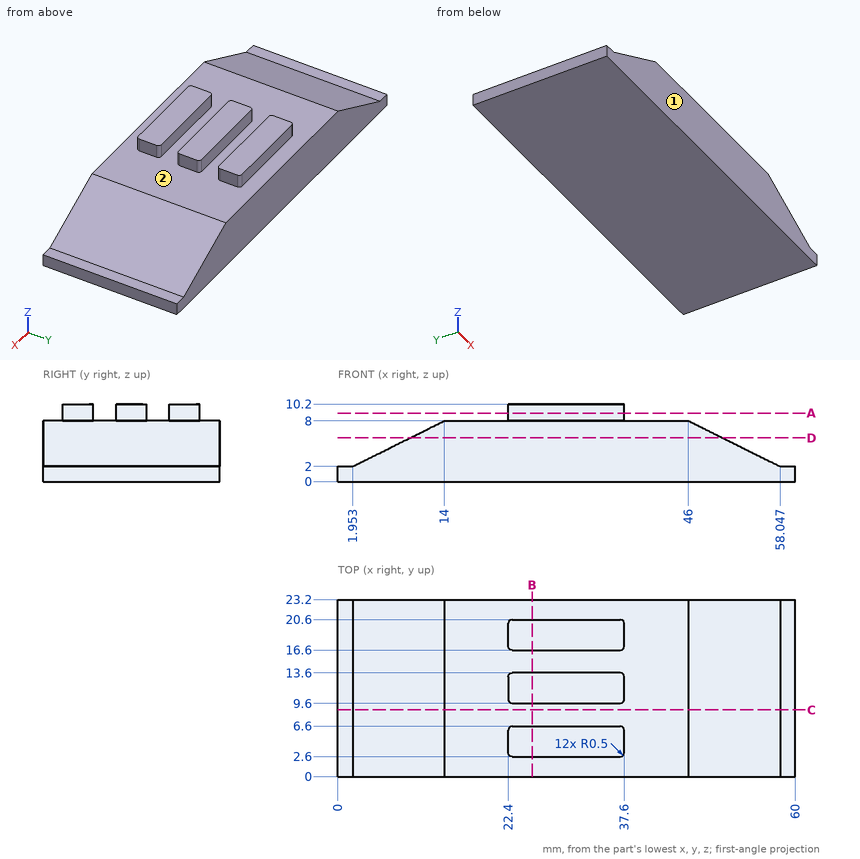
Source: three-view drawing plus pictorial views. Frame: mm from the lowest corner of the part. A direction names the side the tool comes from. Give positions to 0.01 mm unless a question says otherwise; leave off trailing zeros. Order: outer loops, then holes, each group sorted by start corner. A loop starts at its lowest first (then second) coordinate and runs counter-clockwise, first axis right, second up. Notation, with made-up numbers: (52.25, -14.5) -> (75.25, -14.5) arc R34 ccw to (75.25, 20.5) -> close; hole circle Ø1 at (45.25, -3.75). An arc over 180 degrees is marked (long way). Use a Markdown table: item, result.
Q1. Access query for the marked faces 1 and 2. Directions: +Z, -Z, +X, -X, +Y, -Y. A direction counts if a zero-diameter tool reaches every point of the face in a straight line with its end or side. Return the directions, or none.
A:
| item | result |
|---|---|
| face 1 | +Z, -Z, +X, -X, -Y |
| face 2 | +Z |
Q2. Section A-A (z = 9). Return the cut outline in (x, y).
A:
| item | result |
|---|---|
| outline | (22.4, 3.1) arc R0.5 ccw to (22.9, 2.6) -> (37.1, 2.6) arc R0.5 ccw to (37.6, 3.1) -> (37.6, 6.1) arc R0.5 ccw to (37.1, 6.6) -> (22.9, 6.6) arc R0.5 ccw to (22.4, 6.1) -> close; (22.4, 10.1) arc R0.5 ccw to (22.9, 9.6) -> (37.1, 9.6) arc R0.5 ccw to (37.6, 10.1) -> (37.6, 13.1) arc R0.5 ccw to (37.1, 13.6) -> (22.9, 13.6) arc R0.5 ccw to (22.4, 13.1) -> close; (22.4, 17.1) arc R0.5 ccw to (22.9, 16.6) -> (37.1, 16.6) arc R0.5 ccw to (37.6, 17.1) -> (37.6, 20.1) arc R0.5 ccw to (37.1, 20.6) -> (22.9, 20.6) arc R0.5 ccw to (22.4, 20.1) -> close |
Q3. Section D-D (z = 5.75). Return the cut outline in (x, y).
A:
| item | result |
|---|---|
| outline | (9.48, 0) -> (50.52, 0) -> (50.52, 23.2) -> (9.48, 23.2) -> close |
Q4. First-contact query: P1, Ø1.1, axis at y = 11, z = 8.5, coming from the -X side; P2, Ø1.1, axis at x = 29, z = 9, coming from the -Y side; P3, Ø2, axis at x = 14.5, y = 20.5, coming from the +Z side. Flat tips, straight axial feed; report the tip coordinate or a pass-through.
A:
| item | result |
|---|---|
| P1 | x = 13.9 |
| P2 | y = 2.6 |
| P3 | z = 8 |
Q5. Section C-C (y = 8.75). Return the cut outline in (x, z), and give its area (3 significant figures).
A:
| item | result |
|---|---|
| outline | (0, 0) -> (60, 0) -> (60, 2) -> (58.05, 2) -> (46, 8) -> (14, 8) -> (1.95, 2) -> (0, 2) -> close |
| area | 384 mm^2 |
Q6. Material intervals for line 1 (Y direction, x = 37, z = 8.75); line 2 (X direction, y = 17, z = 10); line 3 (Z direction, x = 20.5, y = 5.25), sorted ascending. Write a range as [from, to].
A:
| item | result |
|---|---|
| line 1 | [2.6, 6.6], [9.6, 13.6], [16.6, 20.6] |
| line 2 | [22.41, 37.59] |
| line 3 | [0, 8] |
Q7. Section B-B (x = 25.5). Return the cut outline in (y, z).
A:
| item | result |
|---|---|
| outline | (0, 0) -> (23.2, 0) -> (23.2, 8) -> (20.6, 8) -> (20.6, 10.2) -> (16.6, 10.2) -> (16.6, 8) -> (13.6, 8) -> (13.6, 10.2) -> (9.6, 10.2) -> (9.6, 8) -> (6.6, 8) -> (6.6, 10.2) -> (2.6, 10.2) -> (2.6, 8) -> (0, 8) -> close |
